from build123d import *

# Parameters (mm, degrees)
SKETCH_1_R          = 1
EXTRUDE_1_DEPTH     = 3
CUT_EXTRUDE_1_DEPTH = 3
FILLET_1_R          = 6.35
FILLET_2_R          = 3.81


with BuildPart() as part:
    # 스케치1 → 보스-돌출1 (new body)
    with BuildSketch(Plane.XY):
        with BuildLine():
            ThreePointArc((0.531870722, -10.086704765), (-2.468285539, -6.240741756), (1.193231186, -3.018062075))
            ThreePointArc((1.193231186, -3.018062075), (3.977430532, -3.224017026), (6.736428382, -3.650765557))
            ThreePointArc((6.736428382, -3.650765557), (12.811387699, -5.208096803), (10.373680181, 0.570137648))
            ThreePointArc((10.373680181, 0.570137648), (7.511596171, 2.096172534), (6.79289024, 5.259046091))
            ThreePointArc((6.79289024, 5.259046091), (7.052126243, 11.092699457), (5.26272755, 16.651185512))
            ThreePointArc((5.26272755, 16.651185512), (0.091388125, 19.61858906), (-5.787768566, 20.610431722))
            ThreePointArc((-5.787768566, 20.610431722), (-16.663895396, 18.979214467), (-26.65376361, 14.379916953))
            ThreePointArc((-26.65376361, 14.379916953), (-30.97630157, 10.905433837), (-34.485646455, 6.611150914))
            ThreePointArc((-34.485646455, 6.611150914), (-36.933218927, 1.953038955), (-38.436256849, -3.089727649))
            ThreePointArc((-38.436256849, -3.089727649), (-37.817076352, -4.849129426), (-35.97891327, -5.165413449))
            ThreePointArc((-35.97891327, -5.165413449), (-29.469944847, -4.76402142), (-22.96129319, -5.170517559))
            ThreePointArc((-22.96129319, -5.170517559), (-17.052833669, -5.356485804), (-11.211694851, -4.447874001))
            ThreePointArc((-11.211694851, -4.447874001), (-5.68729426, -7.582685682), (-3.5, -13.546056371))
            ThreePointArc((-3.5, -13.546056371), (2.279084517, -16.20232702), (0.531870722, -10.086704765))
        make_face()
        with Locations((10.16, -2.923333517)):
            Circle(SKETCH_1_R, mode=Mode.SUBTRACT)
        with Locations((0, -13.546056371)):
            Circle(SKETCH_1_R, mode=Mode.SUBTRACT)
    extrude(amount=EXTRUDE_1_DEPTH)

    # 스케치3 → 컷-돌출1 (cut)
    with BuildSketch(Plane.XY.offset(3)):
        Polygon((-37.188543837, -5.783898323), (-34.775495789, -4.001428374), (-36.49557929, -1.672837008), (-38.908627338, -3.455306957), align=None)
        Polygon((-35.300313228, 2.168251474), (-32.945896506, 3.852812812), (-34.691555923, 6.292622886), (-37.045972645, 4.608061549), align=None)
        Polygon((-30.219801903, 8.760975192), (-27.619820697, 10.03420837), (-28.939233317, 12.728489413), (-31.539214523, 11.455256235), align=None)
        Polygon((-22.051978234, 14.155956059), (-19.255706545, 14.905549044), (-20.032486841, 17.803239913), (-22.828758529, 17.053646929), align=None)
        Polygon((-14.526759613, 16.903481061), (-11.645327955, 17.183439276), (-11.935440095, 20.169378818), (-14.816871753, 19.889420603), align=None)
        Polygon((-5.294168633, 20.707213916), (-2.42254789, 20.340036428), (-2.803042696, 17.364263637), (-5.674663439, 17.731441125), align=None)
        Polygon((2.496916602, 18.538725662), (5.307614816, 17.845183627), (4.588918406, 14.932542992), (1.778220193, 15.626085027), align=None)
    extrude(amount=-CUT_EXTRUDE_1_DEPTH, mode=Mode.SUBTRACT)

    # 필렛1
    fillet_1_edges = [part.edges().sort_by_distance(p)[0] for p in [
        (-11.211694851, -4.447874001, 1.5),
    ]]
    fillet(fillet_1_edges, radius=FILLET_1_R)

    # 필렛2
    fillet_2_edges = [part.edges().sort_by_distance(p)[0] for p in [
        (6.736428382, -3.650765557, 1.5),
    ]]
    fillet(fillet_2_edges, radius=FILLET_2_R)


solid = part.part
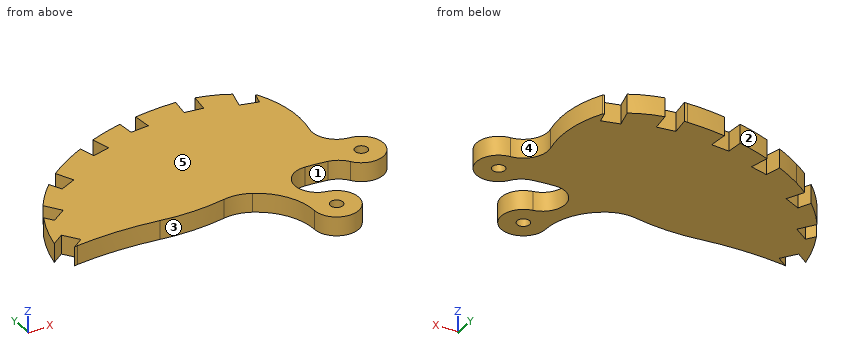
Input: part model. Units: mm. Frame: model coordinates. Face numbers are marked on the shaded views. A direction names the side the tool comes from. Coordinates: 2 decimals unless noted, no trailing zeros. Order: outer loops, then holes, each group sorted by start corner. A loop starts at its lowest first (then second) coordinate and runs counter-clockwise, first axis right, second up. Notation, with made-up numbers: M -40,41.5 L -26,41.5 A9 cw -26,58.5 Z; hole C -9.5,63 d5. An arc over 180 degrees is marked long. Answer in a Markdown table with one row per item.
(1) Section query A-A, the plane x = 0. Output: boundary loops of the cut face in (y, z), plus the area to 3 significant figures.
Numbers:
| item | result |
|---|---|
| outline | M -17.05,0 L -14.55,0 L -14.55,3 L -17.05,3 Z; M -12.55,0 L -9.96,0 L -9.96,3 L -12.55,3 Z; M -3.18,0 L 19.65,0 L 19.65,3 L -3.18,3 Z |
| area | 83.7 mm^2 |
(2) Draft query along X for the marked faces 3, 4 and 5. Return one class per face: pulls with the +X half, pulls with the -X half, needs draft (parallel to the pull), parting line crosses it, or undercut.
Numbers:
| item | result |
|---|---|
| face 3 | undercut |
| face 4 | pulls with the +X half |
| face 5 | needs draft |
(3) Section query C-C, the plane y = 11.5. Output: boundary loops of the cut face in (x, z), plus the area to 3 significant figures.
Numbers:
| item | result |
|---|---|
| outline | M -28.34,0 L 6.99,0 L 6.99,3 L -28.34,3 Z |
| area | 106 mm^2 |
(4) Section query B-B, the plane z = 2.5. Give the number of separate pieces and of enclosed holes in the cut face, plus the area to 3 significant figures.
Numbers:
| item | result |
|---|---|
| separate pieces | 1 |
| enclosed holes | 2 |
| area | 981 mm^2 |
(5) Access query for the marked faces 1 and 2. Directions: +Z, -Z, +X, -X, +Y, -Y. A direction counts if a zero-diameter tool reaches every point of the face in a straight line with its end or side. Return the directions, or none.
Numbers:
| item | result |
|---|---|
| face 1 | +Z, -Z |
| face 2 | +Z, -Z, -X, +Y |
(6) Material intervals for line 1 (Y direction, x = 0, z = 1.7); line 2 (Y direction, x = 10.16, z = 1.8); line 3 (X direction, y = -12, z = 1.75), sorted ascending. Write a range as [from, to].
Numbers:
| item | result |
|---|---|
| line 1 | y = [-17.05, -14.55], [-12.55, -9.96], [-3.18, 19.65] |
| line 2 | y = [-6.42, -3.92], [-1.92, 0.59] |
| line 3 | x = [-3.63, 3.14] |
(7) Section query D-D, the plane x = -15.5. Output: boundary loops of the cut face in (y, z), plus the area to 3 significant figures.
Numbers:
| item | result |
|---|---|
| outline | M -5.22,0 L 19.31,0 L 19.31,3 L -5.22,3 Z |
| area | 73.6 mm^2 |
(8) Contact query for flat-ended pins moving along their axis: pin 1 Ø1 at (x, z) = (-19, 0.5) entering from -Y; pin 2 Ø1 at (x, z) = (-29, 2) entering from +Y; pin 3 Ø1 at (x, z) = (-16, 1) entering from -Y. Output: stop coordinate, or through.
Numbers:
| item | result |
|---|---|
| pin 1 | stops at y = -5.42 |
| pin 2 | stops at y = 13.08 |
| pin 3 | stops at y = -5.32 |
